Part model, mm, in its own coordinate system. Round coordinates to 2 decimals unless told otherwise and drop trailing zeros. Write each loop counter-clockwise with the first axis right and the second up, starting at its lowest first coordinate (ties: lowest second). Pieces come first, ordered by that corner, then holes. Notation, with made-up numbers: M -22,7 L 2,7 A35 cw 2,43 Z; hole C -19.5,49 d4. An arc over 180 degrees is marked long. Use a Markdown table: item, result. Add a question column.
1) Wall check: probe 1 along X at (y, z) = (9.5, 4.5); probe 2 along Y at (x, z) = (1, 4.3); probe 3 along Y at (x, z) = (52.5, 4.8). Give the ranges that are in metal, low to high.
2) Drop flat-ended pins along their axis: P1, Ø1.8, axis at y = 17, z = 3, coming from the +X side; P2, Ø1.8, axis at x = 37.5, z = 2, coming from the -Y side; P3, Ø3, axis at y = 66, z = 4, coming from the +X side. Give the stop position or say it passes through.
3) Slice it at D-D on y = 24. Write the cut outline in (x, z), plus the area to 3 significant figures.
4) Slice it at A-A on y = -23. Write the cut outline in (x, z).
5) Slice it at B-B on z = 3.1. Write the cut outline in (x, y).
6) Slice it at C-C on x = 84. Write the cut outline in (y, z), plus the area to 3 significant figures.
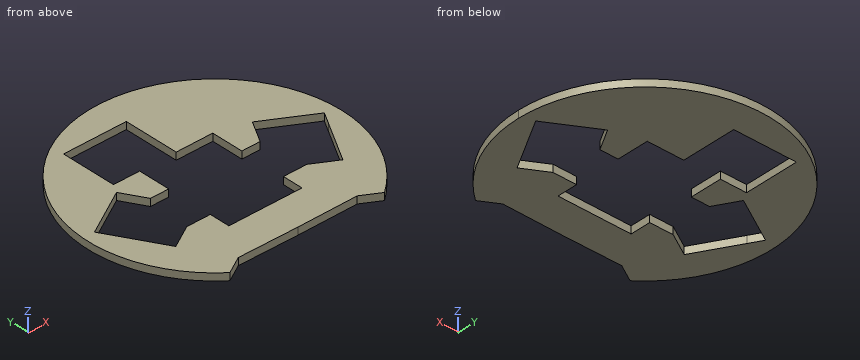
```python
from build123d import *

# Parameters (mm, degrees)
F1_DEPTH = 6


with BuildPart() as f1:
    # F0 (on Top) → F1 (new body)
    with BuildSketch(Plane.XY):
        with BuildLine():
            ThreePointArc((64.075859, -83.182236), (94.215087, -46.352103), (105, 0))
            ThreePointArc((105, 0), (-46.352103, 94.215087), (-64.075859, -83.182236))
            Line((-64.075859, -83.182236), (-49.282032, -74.641016))
            Line((-49.282032, -74.641016), (0, -75))
            Line((0, -75), (49.282032, -74.641016))
            Line((49.282032, -74.641016), (64.075859, -83.182236))
        make_face()
        Polygon((-49.796461, -28.75), (-69.282032, -40), (-89.282032, -5.358984), (-95.282032, 5.033321), (-56.310889, 27.533321), (-45.466334, 8.75), (-30.310889, 8.75), (-30.310889, 35), (-52, 35), (-52, 80), (0, 80), (0, 35), (30.310889, 35), (30.310889, 8.75), (45.466334, 8.75), (56.310889, 27.533321), (95.282032, 5.033321), (89.282032, -5.358984), (69.282032, -40), (49.796461, -28.75), (30.310889, -28.75), (30.310889, -45.5), (-30.310889, -45.5), (-30.310889, -28.75), align=None, mode=Mode.SUBTRACT)
    extrude(amount=F1_DEPTH)


solid = f1.part
```
Entries:
| question | item | result |
|---|---|---|
| 1 | probe 1 | x = -104.57 to -87.55, -45.9 to -30.31, 30.31 to 45.9, 87.55 to 104.57 |
| 1 | probe 2 | y = -74.99 to -45.5, 35 to 105 |
| 1 | probe 3 | y = -76.5 to -30.31, 20.93 to 90.93 |
| 2 | P1 | stops at x = 103.76 |
| 2 | P2 | stops at y = -74.73 |
| 2 | P3 | stops at x = 82.85 |
| 3 | outline | M -102.22,0 L -62.43,0 L -62.43,6 L -102.22,6 Z; M -54.27,0 L -30.31,0 L -30.31,6 L -54.27,6 Z; M 30.31,0 L 54.27,0 L 54.27,6 L 30.31,6 Z; M 62.43,0 L 102.22,0 L 102.22,6 L 62.43,6 Z |
| 3 | area | 765 mm^2 |
| 4 | outline | M -102.45,0 L -79.1,0 L -79.1,6 L -102.45,6 Z; M 79.1,0 L 102.45,0 L 102.45,6 L 79.1,6 Z |
| 5 | outline | M -64.08,-83.18 L -49.28,-74.64 L 0,-75 L 49.28,-74.64 L 64.08,-83.18 A105 ccw 105,0 A105 ccw long Z; hole M -95.28,5.03 L -69.28,-40 L -49.8,-28.75 L -30.31,-28.75 L -30.31,-45.5 L 30.31,-45.5 L 30.31,-28.75 L 49.8,-28.75 L 69.28,-40 L 95.28,5.03 L 56.31,27.53 L 45.47,8.75 L 30.31,8.75 L 30.31,35 L 0,35 L 0,80 L -52,80 L -52,35 L -30.31,35 L -30.31,8.75 L -45.47,8.75 L -56.31,27.53 Z |
| 6 | outline | M -63,0 L -14.51,0 L -14.51,6 L -63,6 Z; M 11.55,0 L 63,0 L 63,6 L 11.55,6 Z |
| 6 | area | 600 mm^2 |
